from build123d import *

# Parameters (mm, degrees)
SKETCH1_W           = 40
SKETCH1_H           = 40
BOSS_EXTRUDE1_DEPTH = 5
SKETCH2_R           = 7.5
BOSS_EXTRUDE2_DEPTH = 5
SKETCH4_R           = 6.225
BOSS_EXTRUDE3_DEPTH = 7
FILLET1_R           = 2.5
SKETCH5_R           = 5
CUT_EXTRUDE1_DEPTH  = 17


with BuildPart() as part:
    # Sketch1 → Boss-Extrude1 (new body)
    with BuildSketch(Plane(origin=(0, 0, 0), x_dir=(1, 0, 0), z_dir=(0, 1, 0))):
        Rectangle(SKETCH1_W, SKETCH1_H)
    extrude(amount=BOSS_EXTRUDE1_DEPTH)

    # Sketch2 → Boss-Extrude2 (add)
    with BuildSketch(Plane(origin=(0, 5, 0), x_dir=(1, 0, 0), z_dir=(0, 1, 0))):
        with Locations(Location((0, 0, 0), (0, 0, 270))):
            Circle(SKETCH2_R)
    extrude(amount=BOSS_EXTRUDE2_DEPTH)

    # Sketch4 → Boss-Extrude3 (add)
    with BuildSketch(Plane(origin=(0, 10, 0), x_dir=(1, 0, 0), z_dir=(0, 1, 0))):
        with Locations(Location((0, 0, 0), (0, 0, 270))):
            Circle(SKETCH4_R)
    extrude(amount=BOSS_EXTRUDE3_DEPTH)

    # Fillet1
    fillet1_edges = [part.edges().sort_by_distance(p)[0] for p in [
        (0, 5, -7.5),
        (20, 2.5, 20),
        (-20, 2.5, 20),
        (-20, 2.5, -20),
        (20, 2.5, -20),
    ]]
    fillet(fillet1_edges, radius=FILLET1_R)

    # Sketch5 → Cut-Extrude1 (cut)
    with BuildSketch(Plane(origin=(0, 17, 0), x_dir=(1, 0, 0), z_dir=(0, 1, 0))):
        with Locations(Location((0, 0, 0), (0, 0, 270))):
            Circle(SKETCH5_R)
    extrude(amount=-CUT_EXTRUDE1_DEPTH, mode=Mode.SUBTRACT)


solid = part.part
Geometry check sheet. Reference: the model listing, model coordinates, mm. A direction names the side the tool comes from. Give positions to 0.01 mm unless a question says otherwise; leave off trailing zeros. Order: outer loops, then holes, each group sorted by start corner. A loop starts at its lowest first (then second) coordinate and runs counter-clockwise, first axis right, second up. Notation, with made-up numbers: (6.5, 5.5) - (52.5, 5.5) arc R9 cw to (52.5, 11.5) - close; hole circle Ø7 at (-2.75, 16.5). An arc over 180 degrees is marked (long way). Answer as a JSON object with one key per item and string values.
(1) Depth check by flat-ended pin: pin 1 Ø8 at (x, y) = (4.5, 13) entering from -Z; pin 2 Ø2 at (x, z) = (-1.5, -12) entering from +Y. Enter the tip coordinate at first touch or a pass-through.
Report:
{"pin 1": "z = -7.27", "pin 2": "y = 5"}
(2) Cross-section at D-D (z = 11.5). Record the cut outline in (x, y).
Report:
{"outline": "(-20, 0) - (20, 0) - (20, 5) - (-20, 5) - close"}
(3) Cross-section at C-C (y = 10.5). Record the cut outline in (x, z) (3 decimals).
Report:
{"outline": "circle Ø12.45 at (0, 0); hole circle Ø10 at (0, 0)"}
(4) Material ranges on line 1 (X direction, y = 7.5, z = 0); line 2 (X direction, y = 12.5, z = 0) (3 decimals); line 3 (Y direction, x = 9.5, z = 16.5), recorded low to high.
Report:
{"line 1": "-7.5 to -5, 5 to 7.5", "line 2": "-6.225 to -5, 5 to 6.225", "line 3": "0 to 5"}
(5) Cross-section at B-B (z = 0). Record the cut outline in (x, y) (3 decimals), then the cut area to 3 significant figures.
Report:
{"outline": "(-20, 0) - (-5, 0) - (-5, 17) - (-6.225, 17) - (-6.225, 10) - (-7.5, 10) - (-7.5, 7.5) arc R2.5 cw to (-10, 5) - (-20, 5) - close; (5, 0) - (20, 0) - (20, 5) - (10, 5) arc R2.5 cw to (7.5, 7.5) - (7.5, 10) - (6.225, 10) - (6.225, 17) - (5, 17) - close", "area": "195 mm^2"}
(6) Tool access check on faces 1 (the flat face through (6, 10, -3)), 2 (the flat face through (20, 2, 0)). Record the directions out of +Z, -Z, +X, -X, +Y, -Y that give a thin tool (end or side, any length) a straight path to the whole face; none if there is none.
Report:
{"face 1": "+Y", "face 2": "+Z, -Z, +X, +Y, -Y"}
(7) Cross-section at A-A (x = 0). Record the cut outline in (y, z) (3 decimals).
Report:
{"outline": "(0, -20) - (5, -20) - (5, -10) arc R2.5 cw to (7.5, -7.5) - (10, -7.5) - (10, -6.225) - (17, -6.225) - (17, -5) - (0, -5) - close; (0, 5) - (17, 5) - (17, 6.225) - (10, 6.225) - (10, 7.5) - (7.5, 7.5) arc R2.5 cw to (5, 10) - (5, 20) - (0, 20) - close"}
(8) Draft check along X on faces 3 (the cylindrical face through (-4.88, 8.62, -1.08)), 4 (the cylindrical face through (-3.79, 13.45, -4.94)), 5 (the flat face through (-5, 0, 4)). Enter one of: released by +X, released by -X, zero draft, split by the parting line, or undercut.
Report:
{"face 3": "undercut", "face 4": "split by the parting line", "face 5": "zero draft"}
